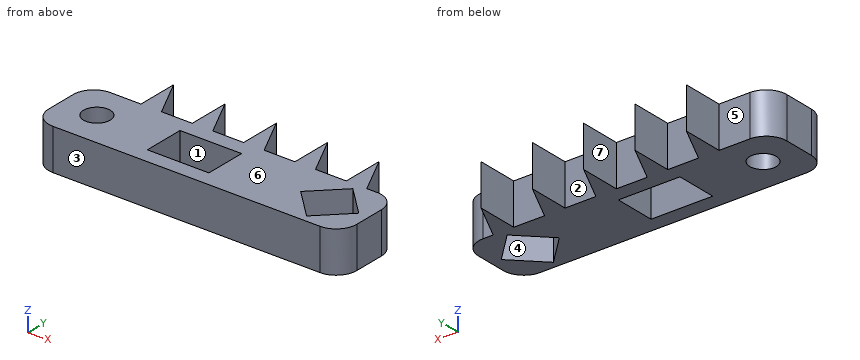
```python
from build123d import *

# Parameters (mm, degrees)
SKETCH_1_R      = 1.3
SKETCH_1_W      = 6
SKETCH_1_H      = 4
EXTRUDE_1_DEPTH = 4
EXTRUDE_2_DEPTH = 4


with BuildPart() as part:
    # Эскиз1 → Бобышка-Вытянуть1 (new body)
    with BuildSketch(Plane.XY):
        with BuildLine():
            Line((2, 0), (28, 0))
            ThreePointArc((28, 0), (29.414213562, 0.585786438), (30, 2))
            Line((30, 2), (30, 5))
            ThreePointArc((30, 5), (29.414213562, 6.414213562), (28, 7))
            Line((28, 7), (2, 7))
            ThreePointArc((2, 7), (0.585786438, 6.414213562), (0, 5))
            Line((0, 5), (0, 2))
            ThreePointArc((0, 2), (0.585786438, 0.585786438), (2, 0))
        make_face()
        with Locations((3.5, 3.5)):
            Circle(SKETCH_1_R, mode=Mode.SUBTRACT)
        Polygon((23.343145751, 3.5), (26.171572875, 6.328427125), (29, 3.5), (26.171572875, 0.671572875), align=None, mode=Mode.SUBTRACT)
        with Locations((13, 3.5)):
            Rectangle(SKETCH_1_W, SKETCH_1_H, mode=Mode.SUBTRACT)
    extrude(amount=EXTRUDE_1_DEPTH)

    # Эскиз2 → Бобышка-Вытянуть2 (add)
    with BuildSketch(Plane.XY.offset(4)):
        Polygon((5, 7), (5, 11), (7, 7), align=None)
        Polygon((10, 7), (10, 11), (12, 7), align=None)
        Polygon((15, 7), (15, 11), (17, 7), align=None)
        Polygon((20, 7), (20, 11), (22, 7), align=None)
        Polygon((25, 7), (25, 11), (27, 7), align=None)
    extrude(amount=-EXTRUDE_2_DEPTH)


solid = part.part
```
Part model, mm, in its own coordinate system. Face numbers are marked on the shaded views. A direction names the side the tool comes from. Round coordinates to 2 decimals unless told otherwise and drop trailing zeros. Loops run counter-clockwise (first coordinate to the right, second up) from the corner with the lowest first, then second, coordinate; pieces in that order, holes last.
1. Slice it at B-B (z = 3). Count the separate pieces of the cut face and the enclosed holes in it, and give its area (3 significant figures).
Solutions:
separate pieces: 1
enclosed holes: 3
area: 181 mm2
2. Flat gauge pins, fed straight in: pin 1 (1.5 mm diameter, centred on x = 4, z = 2.5, fed in from +Y); pin 2 (2 mm diameter, centred on y = 9.5, z = 3, fed in from -X); pin 3 (1.5 mm diameter, centred on x = 14, y = 8, fed in from +Z). Where does each tip first touch, or does it go through?
Solutions:
pin 1: stops at y = 7
pin 2: stops at x = 5
pin 3: passes through
3. 3-axis set-ups, long thin cutter, end or side, ignore diameter. For the marked faces 5, 6 and 7: which of +Z, -Z, +X, -X, +Y, -Y reach the whole face in a straight line?
Solutions:
face 5: +Z, -Z, -X, +Y
face 6: +Z, +X, -X, +Y, -Y
face 7: +Z, -Z, +Y
4. Drill centre lines: line 1 along Y through (x, z) = (14.25, 0.9); line 2 along Y through (x, z) = (3.5, 3); line 3 along X through (y, z) = (2.75, 2.1). Where is each one in solid material? Low to high.
Solutions:
line 1: y = 0 to 1.5, 5.5 to 7
line 2: y = 0 to 2.2, 4.8 to 7
line 3: x = 0 to 2.44, 4.56 to 10, 16 to 24.09, 28.25 to 30
5. Slice it at C-C (y = 10). Give the cut face in (x, z), and give its area (3 significant figures).
Solutions:
outline: (5, 0) - (5.5, 0) - (5.5, 4) - (5, 4) - close; (10, 0) - (10.5, 0) - (10.5, 4) - (10, 4) - close; (15, 0) - (15.5, 0) - (15.5, 4) - (15, 4) - close; (20, 0) - (20.5, 0) - (20.5, 4) - (20, 4) - close; (25, 0) - (25.5, 0) - (25.5, 4) - (25, 4) - close
area: 10.0 mm2
6. Slice it at D-D (x = 7.5). Give the cut face in (y, z), and give its area (3 significant figures).
Solutions:
outline: (0, 0) - (7, 0) - (7, 4) - (0, 4) - close
area: 28.0 mm2
7. Two-plate mould, pull along Y, no slides. Class the marked faces 1, 2, 3 and 4: pulls with the +Y half, pulls with the -Y half, needs draft (parallel to the pull), parting line crosses it, or undercut.
Solutions:
face 1: undercut
face 2: pulls with the +Y half
face 3: pulls with the -Y half
face 4: undercut
8. Slice it at A-A (x = 3.5). Give the cut face in (y, z).
Solutions:
outline: (0, 0) - (2.2, 0) - (2.2, 4) - (0, 4) - close; (4.8, 0) - (7, 0) - (7, 4) - (4.8, 4) - close
